Model file for the job. Use its own axes, mm. A direction names the side the tool comes from. Round coordinates to 2 decimals unless told otherwise and drop trailing zeros. Use a Markdown table: item, result. Add a question column.
Q1. Pin check, flat tips, straight feed: pin 1 (12 mm diameter, centred on y = -13.5, z = 22, fed in from -X); pin 2 (2 mm diameter, centred on x = -38.5, z = 21.5, fed in from -Y); pin 3 (2.5 mm diameter, centred on y = -11.5, z = 3, fed in from +X); pin 4 (2.5 mm diameter, centred on x = -30.5, y = -7, fed in from +Z). Stop position of each tip, or through.
Q2. Probe line 1 (Y direction, x = -25, z = 3.75); line 2 (Y direction, x = -13.5, z = 8.5); line 3 (Y direction, x = -22, z = 1.25). List the from-to ranges inside material, lowest first. Write a range as from..to.
Q3. Cut at A-A (z = 3). State how many separate pieces and enclosed holes the cut face has, plus the area to 3 significant figures.
Q4. Mould opens along X. For faces 5 (the face through (-29.38, -17.59, 4.36)), 6 (the face through (-29, -9.883, 5)), 7 (the face through (-29, 18.916, 10)) say: +X half, -X half, draft (parallel to the pull), parting line (faces both ways), or undercut.
Q5. Tool access for faces 1 (the face through (-29.3, -12.3, 2.3)), 2 (the face through (-34.582, -11, 3)), 3 (the face through (-29, -4.383, 9)), 4 (the face through (-29, -12.883, 5)): list every direction of +Z, -Z, +X, -X, +Y, -Y with a clear straight run to the whole face (end or side of a thin tool).
from build123d import *

# Parameters (mm, degrees)
REVOLUCI_N1_ANGLE     = 180
CROQUIS2_W            = 2
CROQUIS2_H            = 3
CORTAR_EXTRUIR1_DEPTH = 15
CORTAR_EXTRUIR2_START = -6.6
CROQUIS3_W            = 7.076217781
CROQUIS3_H            = 3
CROQUIS3_W_2          = 6.688868885
CORTAR_EXTRUIR2_DEPTH = 6.6


with BuildPart() as part:
    # Croquis1 → Revolución1 (revolve)
    with BuildSketch(Plane.XY):
        with BuildLine():
            Line((-51.782166939, -4.382597623), (-31.582166939, -4.382597623))
            Line((-31.582166939, -4.382597623), (-31.582166939, -19.966657293))
            Line((-31.582166939, -19.966657293), (-36.798543174, -13.956174379))
            Line((-36.798543174, -13.956174379), (-36.798543174, -5.882597623))
            Line((-36.798543174, -5.882597623), (-43.248543174, -5.882597623))
            Line((-43.248543174, -5.882597623), (-53.282166939, -5.882597623))
            ThreePointArc((-53.282166939, -5.882597623), (-56.573748762, 6.516780598), (-53.282166939, 18.916158819))
            Line((-53.282166939, 18.916158819), (-29.282166939, 18.916158819))
            Line((-29.282166939, 18.916158819), (-29.282166939, 17.416158819))
            Line((-29.282166939, 17.416158819), (-51.782166939, 17.416158819))
            ThreePointArc((-51.782166939, 17.416158819), (-54.283199087, 6.516780598), (-51.782166939, -4.382597623))
        make_face()
    revolve(axis=Axis((-29.282166939, 17.416158819, 0), (0, 1, 0)), revolution_arc=REVOLUCI_N1_ANGLE)

    # Croquis2 → Cortar-Extruir1 (cut)
    with BuildSketch(Plane(origin=(0, 0, 0), x_dir=(-1, 0, 0), z_dir=(0, 0, -1))):
        with Locations((24.982166939, -7.382597623)):
            Rectangle(CROQUIS2_W, CROQUIS2_H)
        with Locations((33.582166939, -7.382597623)):
            Rectangle(CROQUIS2_W, CROQUIS2_H)
        with Locations((33.582166939, -11.382597623)):
            Rectangle(CROQUIS2_W, CROQUIS2_H)
        with Locations((24.982166939, -11.382597623)):
            Rectangle(CROQUIS2_W, CROQUIS2_H)
    extrude(amount=-CORTAR_EXTRUIR1_DEPTH, mode=Mode.SUBTRACT)

    # Croquis3 → Cortar-Extruir2 (cut)
    with BuildSketch(Plane.ZY.offset(32.582166939).offset(CORTAR_EXTRUIR2_START)):
        with Locations((8.321249271, -11.382597623)):
            Rectangle(CROQUIS3_W, CROQUIS3_H)
        with Locations((8.127574822, -7.382597623)):
            Rectangle(CROQUIS3_W_2, CROQUIS3_H)
    extrude(amount=CORTAR_EXTRUIR2_DEPTH, mode=Mode.SUBTRACT)


solid = part.part
Checked values:
| question | item | result |
|---|---|---|
| 1 | pin 1 | passes through |
| 1 | pin 2 | stops at y = -5.88 |
| 1 | pin 3 | stops at x = -21.97 |
| 1 | pin 4 | stops at z = 24.05 |
| 2 | line 1 | y = -16.06..-12.88, -9.88..-8.88, -5.88..-4.38, 17.42..18.92 |
| 2 | line 2 | y = -5.88..-4.38, 17.42..18.92 |
| 2 | line 3 | y = -14.1..-4.38, 17.42..18.92 |
| 3 | separate pieces | 1 |
| 3 | enclosed holes | 5 |
| 3 | area | 377 mm^2 |
| 4 | face 5 | parting line |
| 4 | face 6 | undercut |
| 4 | face 7 | draft |
| 5 | face 1 | -Z, -Y |
| 5 | face 2 | +Z, -Z |
| 5 | face 3 | -Z |
| 5 | face 4 | +Z |
